from build123d import *

# Parameters (mm, degrees)
SKETCH1_W           = 242.82
SKETCH1_H           = 287.3
BOSS_EXTRUDE1_DEPTH = 6.35
SKETCH4_W           = 255.52
SKETCH4_H           = 300
BOSS_EXTRUDE4_DEPTH = 6.4008
SKETCH5_W           = 242.82
SKETCH5_H           = 2.54
BOSS_EXTRUDE5_DEPTH = 49.5808
LPATTERN1_COUNT     = 21
LPATTERN1_PITCH     = 12.7


with BuildPart() as part:
    # Sketch1 → Boss-Extrude1 (new body)
    with BuildSketch(Plane(origin=(0, 0, 0), x_dir=(1, 0, 0), z_dir=(0, 1, 0))):
        Rectangle(SKETCH1_W, SKETCH1_H)
    extrude(amount=-BOSS_EXTRUDE1_DEPTH)

    # Sketch4 → Boss-Extrude4 (add)
    with BuildSketch(Plane(origin=(0, 0, 0), x_dir=(1, 0, 0), z_dir=(0, 1, 0))):
        Rectangle(SKETCH4_W, SKETCH4_H)
    extrude(amount=BOSS_EXTRUDE4_DEPTH)


with BuildPart() as body_2:
    # Sketch5 → Boss-Extrude5 (new body)
    with BuildSketch(Plane.XZ.offset(6.35)):
        with Locations((0, 129.68)):
            Rectangle(SKETCH5_W, SKETCH5_H)
    boss_extrude5 = extrude(amount=-BOSS_EXTRUDE5_DEPTH)


with BuildPart() as lpattern1_1:
    # LPattern1: pattern copy
    add(boss_extrude5.moved(Location(Vector(0, 0, -1) * (1 * LPATTERN1_PITCH))))


with BuildPart() as lpattern1_2:
    # LPattern1: pattern copy
    add(boss_extrude5.moved(Location(Vector(0, 0, -1) * (2 * LPATTERN1_PITCH))))


with BuildPart() as lpattern1_3:
    # LPattern1: pattern copy
    add(boss_extrude5.moved(Location(Vector(0, 0, -1) * (3 * LPATTERN1_PITCH))))


with BuildPart() as lpattern1_4:
    # LPattern1: pattern copy
    add(boss_extrude5.moved(Location(Vector(0, 0, -1) * (4 * LPATTERN1_PITCH))))


with BuildPart() as lpattern1_5:
    # LPattern1: pattern copy
    add(boss_extrude5.moved(Location(Vector(0, 0, -1) * (5 * LPATTERN1_PITCH))))


with BuildPart() as lpattern1_6:
    # LPattern1: pattern copy
    add(boss_extrude5.moved(Location(Vector(0, 0, -1) * (6 * LPATTERN1_PITCH))))


with BuildPart() as lpattern1_7:
    # LPattern1: pattern copy
    add(boss_extrude5.moved(Location(Vector(0, 0, -1) * (7 * LPATTERN1_PITCH))))


with BuildPart() as lpattern1_8:
    # LPattern1: pattern copy
    add(boss_extrude5.moved(Location(Vector(0, 0, -1) * (8 * LPATTERN1_PITCH))))


with BuildPart() as lpattern1_9:
    # LPattern1: pattern copy
    add(boss_extrude5.moved(Location(Vector(0, 0, -1) * (9 * LPATTERN1_PITCH))))


with BuildPart() as lpattern1_10:
    # LPattern1: pattern copy
    add(boss_extrude5.moved(Location(Vector(0, 0, -1) * (10 * LPATTERN1_PITCH))))


with BuildPart() as lpattern1_11:
    # LPattern1: pattern copy
    add(boss_extrude5.moved(Location(Vector(0, 0, -1) * (11 * LPATTERN1_PITCH))))


with BuildPart() as lpattern1_12:
    # LPattern1: pattern copy
    add(boss_extrude5.moved(Location(Vector(0, 0, -1) * (12 * LPATTERN1_PITCH))))


with BuildPart() as lpattern1_13:
    # LPattern1: pattern copy
    add(boss_extrude5.moved(Location(Vector(0, 0, -1) * (13 * LPATTERN1_PITCH))))


with BuildPart() as lpattern1_14:
    # LPattern1: pattern copy
    add(boss_extrude5.moved(Location(Vector(0, 0, -1) * (14 * LPATTERN1_PITCH))))


with BuildPart() as lpattern1_15:
    # LPattern1: pattern copy
    add(boss_extrude5.moved(Location(Vector(0, 0, -1) * (15 * LPATTERN1_PITCH))))


with BuildPart() as lpattern1_16:
    # LPattern1: pattern copy
    add(boss_extrude5.moved(Location(Vector(0, 0, -1) * (16 * LPATTERN1_PITCH))))


with BuildPart() as lpattern1_17:
    # LPattern1: pattern copy
    add(boss_extrude5.moved(Location(Vector(0, 0, -1) * (17 * LPATTERN1_PITCH))))


with BuildPart() as lpattern1_18:
    # LPattern1: pattern copy
    add(boss_extrude5.moved(Location(Vector(0, 0, -1) * (18 * LPATTERN1_PITCH))))


with BuildPart() as lpattern1_19:
    # LPattern1: pattern copy
    add(boss_extrude5.moved(Location(Vector(0, 0, -1) * (19 * LPATTERN1_PITCH))))


with BuildPart() as lpattern1_20:
    # LPattern1: pattern copy
    add(boss_extrude5.moved(Location(Vector(0, 0, -1) * (20 * LPATTERN1_PITCH))))


with BuildPart() as part_1:
    add(part.part)

    # Combine1: cut body 2, LPattern1_1, LPattern1_2, LPattern1_3, LPattern1_5, LPattern1_6, LPattern1_4, LPattern1_7, LPattern1_8, LPattern1_10, LPattern1_11, LPattern1_9, LPattern1_12, LPattern1_16, LPattern1_18, LPattern1_20, LPattern1_19, LPattern1_17, LPattern1_15, LPattern1_14, LPattern1_13
    add(body_2.part, mode=Mode.SUBTRACT)
    add(lpattern1_1.part, mode=Mode.SUBTRACT)
    add(lpattern1_2.part, mode=Mode.SUBTRACT)
    add(lpattern1_3.part, mode=Mode.SUBTRACT)
    add(lpattern1_5.part, mode=Mode.SUBTRACT)
    add(lpattern1_6.part, mode=Mode.SUBTRACT)
    add(lpattern1_4.part, mode=Mode.SUBTRACT)
    add(lpattern1_7.part, mode=Mode.SUBTRACT)
    add(lpattern1_8.part, mode=Mode.SUBTRACT)
    add(lpattern1_10.part, mode=Mode.SUBTRACT)
    add(lpattern1_11.part, mode=Mode.SUBTRACT)
    add(lpattern1_9.part, mode=Mode.SUBTRACT)
    add(lpattern1_12.part, mode=Mode.SUBTRACT)
    add(lpattern1_16.part, mode=Mode.SUBTRACT)
    add(lpattern1_18.part, mode=Mode.SUBTRACT)
    add(lpattern1_20.part, mode=Mode.SUBTRACT)
    add(lpattern1_19.part, mode=Mode.SUBTRACT)
    add(lpattern1_17.part, mode=Mode.SUBTRACT)
    add(lpattern1_15.part, mode=Mode.SUBTRACT)
    add(lpattern1_14.part, mode=Mode.SUBTRACT)
    add(lpattern1_13.part, mode=Mode.SUBTRACT)


solid = part_1.part
Input: part model. Units: mm. Frame: model coordinates. A direction names the side the tool comes from. Coordinates: 2 decimals unless noted, no trailing zeros. Write each loop counter-clockwise with the first axis right and the second up, starting at its lowest first coordinate (ties: lowest second). Pieces come first, ordered by that corner, then holes. Notation, with made-up numbers: M 32.25,41.5 L 60.25,41.5 A19 cw 60.25,57.5 Z; hole C 2.5,75.5 d10. An arc over 180 degrees is marked long. Answer as a JSON object with one key per item and string values. Group by question number.
(1) Contact query for flat-ended pins moving along their axis: P1, Ø2, axis at x = 66, z = -72.5, coming from the +Y side; P2, Ø3, axis at x = 84.5, y = -4, coming from the -Z side; P3, Ø5, axis at y = -3.5, z = -16.5, coming from the -X side. Output: stop coordinate, or through.
(2) Set-up query: faces 1 (the face through (-2, -6.35, 9)), 2 (the face through (-121.41, -3, 111)), 3 (the face through (-2, 3, -150)), 4 (the face through (-2, 0, 90.31)), 5 (the face through (121.41, -3, 98)). Return all of +Z, -Z, +X, -X, +Y, -Y with unobstructed straight access to the full face (end or side cutting, diameter ignored); none if empty.
(3) Section B-B on x = -63. Give the number of separate pieces and of enclosed holes in the cut face, plus the area to 3 significant figures.
(4) Section A-A on z = -28.5. Output: boundary loops of the cut face in (x, y), plus the area to 3 significant figures.
(5) Ray query, line 1 along X through (y, z) = (3.5, 3); line 2 along X through (y, z) = (-2.25, -14). Return the intervals inside material, ascending. Write a range as [from, to].
Result set:
{
 "1": {"P1": "stops at y = 6.4", "P2": "stops at z = -143.65", "P3": "stops at x = -121.41"},
 "2": {"face 1": "+Z, -Z, +X, -X, -Y", "face 2": "+Z, -Z, -X, -Y", "face 3": "-Z, +X, -X, +Y, -Y", "face 4": "+Y, -Y", "face 5": "+Z, -Z, +X, -Y"},
 "3": {"separate pieces": "22", "enclosed holes": "0", "area": "3,060 mm2"},
 "4": {"outline": "M -127.76,0 L -121.41,0 L -121.41,-6.35 L 121.41,-6.35 L 121.41,0 L 127.76,0 L 127.76,6.4 L -127.76,6.4 Z", "area": "3,180 mm2"},
 "5": {"line 1": "x = [-127.76, -121.41], [121.41, 127.76]", "line 2": "x = [-121.41, 121.41]"}
}
